Can you work these out from the drawing? Everything is in mm from the part's minimum corner. A direction names the side the tool comes from. Coordinates: 2 decimals unless noted, no trailing zeros. Loops run counter-clockwise (first coordinate to the right, second up) from the corner with the lowest first, then second, coordinate; pieces in that order, holes last. Notation, with made-up numbers: (15, 30.25) - (54, 30.25) arc R10 cw to (54, 39.25) - close; hole circle Ø6 at (15, 6.25). An arc over 180 degrees is marked (long way). One line per question, with ' | ' between items. Start each with the question number.
1. Which directions (+Z, -Z, +X, -X, +Y, -Y) give clear straight access to the entire face, cutting with the end or side of a thin tool? Please do the marked faces 1, 2 and 3.
2. We'd pull the mould along X, two halves only. Please class the marked faces 4, 5 and 6: pulls with the +X half, pulls with the -X half, needs draft (parallel to the pull), parting line crosses it, or undercut.
3. I'm going to push flat-ended pins straight in: P1, Ø1.5, axis at x = 97, y = 15, coming from the +Z side; P2, Ø6, axis at y = 7, z = 102.5, coming from the -X side; P3, Ø10, axis at x = 129.5, y = 16.5, coming from the -Z side. Where does each tip first touch, or does it pass through?
4. I want a section at B-B, the plane y = 8.5. Write out the boundary of the cut face in (x, z) (1 decimal), then the cut area to 3 significant figures.
5. Please list where these lines run through material, in increasing order: L1, parallel to Y at x = 126.5, z = 160; L2, parallel to X at y = 18, z = 90 (1 decimal); L3, parallel to X at y = 6.75, z = 91.5 (1 decimal). Write a range as [from, to].
6. I want a section at C-C, the plane z = 86.5. Write out the boundary of the cut face in (x, y) (1 decimal).
7. I want a section at D-D, the plane x = 117.5. Write out the boundary of the cut face in (y, z), then the cut area to 3 significant figures.
8. I want a section at A-A, the plane x = 85. Write out the boundary of the cut face in (y, z).
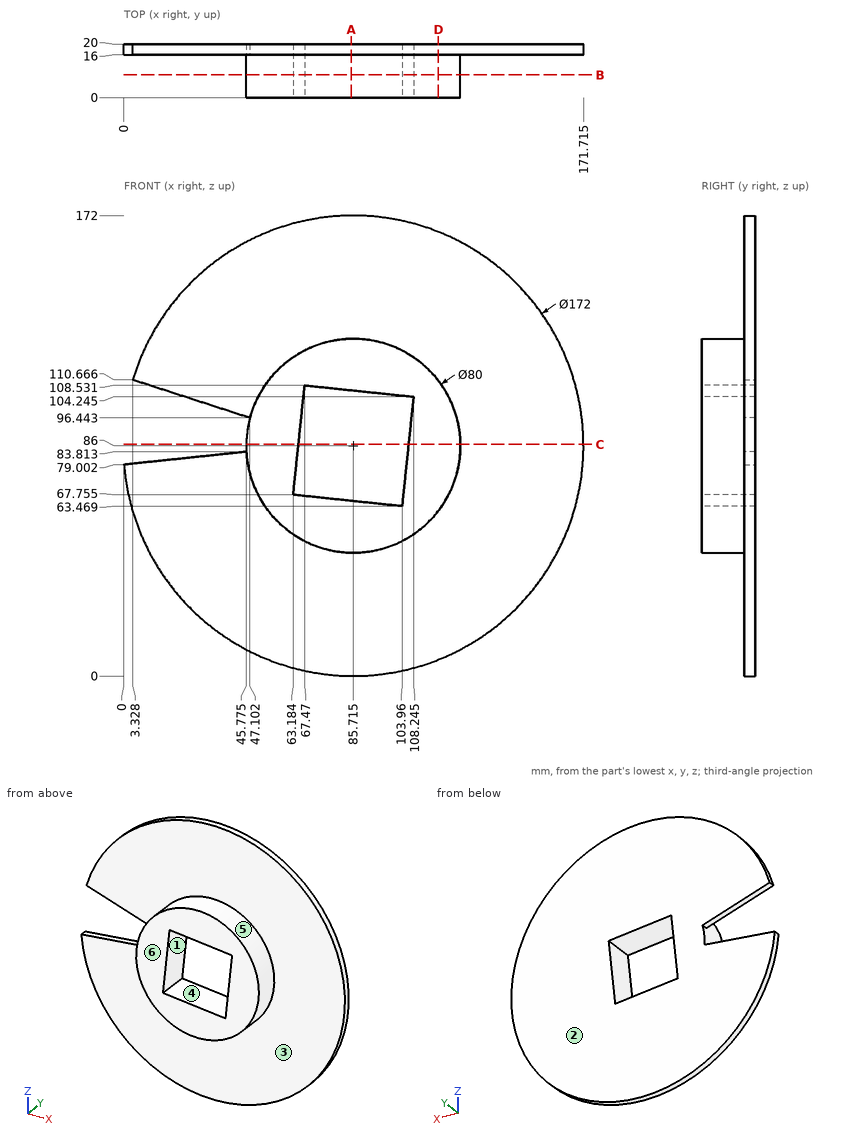
Results are:
1) face 1: +Y, -Y | face 2: +Z, -Z, +X, -X, +Y | face 3: -Y
2) face 4: undercut | face 5: parting line crosses it | face 6: needs draft
3) P1: stops at z = 124.59 | P2: stops at x = 48.06 | P3: stops at z = 9.24
4) outline: circle Ø80 at (85.7, 86); hole (63.2, 67.8) - (104, 63.5) - (108.2, 104.2) - (67.5, 108.5) - close | area: 3,350 mm2
5) L1: y = [16, 20] | L2: x = [45.9, 65.5], [106.7, 171.6] | L3: x = [46.1, 65.7], [106.9, 125.3]
6) outline: (45.7, 0) - (65.2, 0) - (65.2, 20) - (45.7, 20) - close; (106.4, 0) - (125.7, 0) - (125.7, 16) - (171.7, 16) - (171.7, 20) - (106.4, 20) - close
7) outline: (0, 61.72) - (16, 61.72) - (16, 6.09) - (20, 6.09) - (20, 165.91) - (16, 165.91) - (16, 110.28) - (0, 110.28) - close | area: 1,420 mm2
8) outline: (0, 46.01) - (16, 46.01) - (16, 0) - (20, 0) - (20, 65.46) - (0, 65.46) - close; (0, 106.69) - (20, 106.69) - (20, 172) - (16, 172) - (16, 125.99) - (0, 125.99) - close
